from build123d import *

# Parameters (mm, degrees)
F0_R     = 10
F1_DEPTH = 285
F2_R     = 6
F3_DEPTH = 25
F4_R     = 5
F5_DEPTH = 50


with BuildPart() as f1:
    # F0 (on Front) → F1 (new body)
    with BuildSketch(Plane.XZ):
        Circle(F0_R)
    extrude(amount=F1_DEPTH)

    # F2 (on face) → F3 (cut)
    with BuildSketch(Plane.XZ.offset(285)):
        Circle(F2_R)
    extrude(amount=-F3_DEPTH, mode=Mode.SUBTRACT)

    # F4 (on face) → F5 (join)
    with BuildSketch(Plane(origin=(0, 0, 0), x_dir=(-1, 0, 0), z_dir=(0, 1, 0))):
        Circle(F4_R)
    extrude(amount=F5_DEPTH)


solid = f1.part
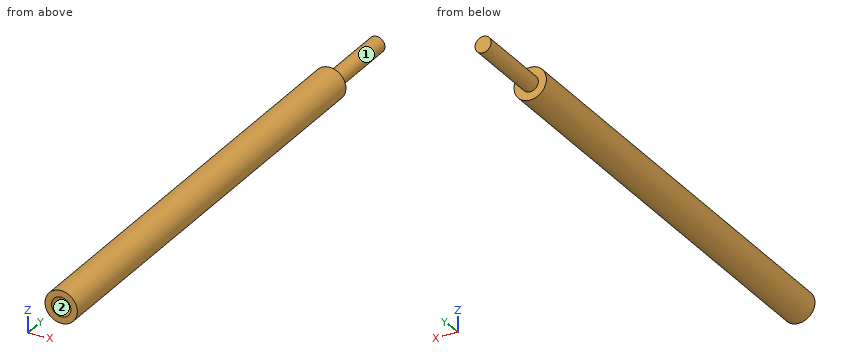
The listing builds one solid part. Answer for the finished solid, in the listing's coordinates (mm). Face numbers are marked on the shaded views. Coordinates: 2 decimals unless noted, no trailing zeros. Loops run counter-clockwise (first coordinate to the right, second up) from the corner with the lowest first, then second, coordinate; pieces in that order, holes last.
1) Flat-ended cylindrical pins translate along their axes: pin 1 Ø1.5 at (y, z) = (-13.5, 3.5) entering from -X; pin 2 Ø9.5 at (x, z) = (2, 1) entering from -Y; pin 3 Ø4 at (x, y) = (5, -143) entering from +Z; pin 4 Ø1 at (y, z) = (-98, -7) entering from +X. Find the tip coordinate at first contact, or state that the pin passes through.
2) Find section B-B on x = 0. Write down the section's boundary in (y, z), then the cut area to 3 significant figures.
3) Find the intervals of material crossed by L1, parallel to Z at x = 0, y = -277; L2, parallel to Y at x = -5.5, z = 5.25; L3, parallel to Y at x = 3.25, z = 3.75, in increasing order.
4) Determine the mould class of the marked faces 1 and 2 for opening direction X: pulls with the +X half, pulls with the -X half, needs draft (parallel to the pull), parting line crosses it, or undercut.
5) Find section A-A on z = 0. Write down the section's boundary in (x, y), then the cut area to 3 significant figures.
6) Find section C-C on y = -20.5. Write down the section's boundary in (x, z).
Values:
1. pin 1: stops at x = -9.61
1. pin 2: stops at y = -285
1. pin 3: stops at z = 9.54
1. pin 4: stops at x = 7.6
2. outline: (-285, -10) - (0, -10) - (0, -5) - (50, -5) - (50, 5) - (0, 5) - (0, 10) - (-285, 10) - (-285, 6) - (-260, 6) - (-260, -6) - (-285, -6) - close
2. area: 5,900 mm2
3. L1: z = -10 to -6, 6 to 10
3. L2: y = -285 to 0
3. L3: y = -260 to 50
4. face 1: parting line crosses it
4. face 2: undercut
5. outline: (-10, -285) - (-6, -285) - (-6, -260) - (6, -260) - (6, -285) - (10, -285) - (10, 0) - (5, 0) - (5, 50) - (-5, 50) - (-5, 0) - (-10, 0) - close
5. area: 5,900 mm2
6. outline: circle Ø20 at (0, 0)
